Geometry check sheet. Reference: the model listing, model coordinates, mm. Face numbers are marked on the shaded views. A direction names the side the tool comes from. Coordinates: 2 decimals unless noted, no trailing zeros. Write each loop counter-clockwise with the first axis right and the second up, starting at its lowest first coordinate (ties: lowest second). Pieces come first, ordered by that corner, then holes. Notation, with made-up numbers: (-12.5, 75) -> (18.5, 75) arc R7 cw to (18.5, 84) -> close; hole circle Ø5 at (-6.5, -8). An arc over 180 degrees is marked (long way). One line per question, with ' | ' between items.
```python
from build123d import *

# Parameters (mm, degrees)
CUT_EXTRUDE1_DEPTH                 = 65.668384857
CHAMFER1_SIZE                      = 0.34
SOCKET_HEAD_CAP_SCREW1_D           = 6
SOCKET_HEAD_CAP_SCREW1_CBORE_D     = 9.5
SOCKET_HEAD_CAP_SCREW1_CBORE_DEPTH = 6
CUT_EXTRUDE2_DEPTH                 = 45
BOSS_EXTRUDE1_DEPTH                = 5
SKETCH7_R                          = 1.5
BOSS_EXTRUDE2_DEPTH                = 1
REVOLVE3_ANGLE                     = 90
REVOLVE4_ANGLE                     = 90
TAP1_START                         = 4.7999999
TAP1_OUTLINE_R                     = 2.4585
TAP1_DEPTH                         = 7.2000001


# Read off the part's stored shape, not the designer's step: Tap1
with BuildPart() as part:
    # Sketch1 → Revolve1 (revolve)
    with BuildSketch(Plane.XY, mode=Mode.PRIVATE) as revolve1_sk:
        Polygon((0, 29), (12, 29), (12, 7.5), (-50, 7.5), (-50, 17), (-0.8, 17), (-0.8, 16.32), (0, 16.32), align=None)
    revolve(revolve1_sk.sketch.rotate(Axis((-50, 0, 0), (1, 0, 0)), 90), axis=Axis((-50, 0, 0), (1, 0, 0)))

    # Sketch2 → Cut-Extrude1 (cut, through all)
    with BuildSketch(Plane(origin=(0, 0, 0), x_dir=(0, 0, -1), z_dir=(1, 0, 0))):
        with BuildLine():
            Line((14.696938457, 25), (-14.696938457, 25))
            ThreePointArc((-14.696938457, 25), (0, 29), (14.696938457, 25))
        make_face()
        with BuildLine():
            Line((17, 23.494680249), (17, -23.494680249))
            ThreePointArc((17, -23.494680249), (29, 0), (17, 23.494680249))
        make_face()
        with BuildLine():
            Line((14.696938457, -25), (-14.696938457, -25))
            ThreePointArc((-14.696938457, -25), (0, -29), (14.696938457, -25))
        make_face()
        with BuildLine():
            Line((-17, -23.494680249), (-17, 23.494680249))
            ThreePointArc((-17, 23.494680249), (-29, 0), (-17, -23.494680249))
        make_face()
    extrude(amount=CUT_EXTRUDE1_DEPTH, mode=Mode.SUBTRACT)

    # Chamfer1
    chamfer1_edges = [part.edges().sort_by_distance(p)[0] for p in [
        (-50, 0, -17),
    ]]
    chamfer(chamfer1_edges, length=CHAMFER1_SIZE)

    # Socket Head Cap Screw1 (through all)
    with Locations(Plane(origin=(12, 0, 0), x_dir=(0, 0, -1), z_dir=(1, 0, 0))):
        with Locations((-11.25, 19.485571585), (11.25, -19.485571585), (-11.25, -19.485571585), (11.25, 19.485571585)):
            CounterBoreHole(SOCKET_HEAD_CAP_SCREW1_D / 2, SOCKET_HEAD_CAP_SCREW1_CBORE_D / 2, SOCKET_HEAD_CAP_SCREW1_CBORE_DEPTH)

    # Sketch5 → Cut-Extrude2 (cut)
    with BuildSketch(Plane(origin=(0, 0, 0), x_dir=(0, 0, -1), z_dir=(1, 0, 0))):
        with BuildLine():
            Line((-11, -12.961481397), (-11, 12.961481397))
            ThreePointArc((-11, 12.961481397), (-17, 0), (-11, -12.961481397))
        make_face()
    extrude(amount=-CUT_EXTRUDE2_DEPTH, mode=Mode.SUBTRACT)

    # Sketch6 → Boss-Extrude1 (add)
    with BuildSketch(Plane(origin=(0, 0, 11), x_dir=(-1, 0, 0), z_dir=(0, 0, -1))):
        with BuildLine():
            Line((6.5, 4), (36, 4))
            ThreePointArc((36, 4), (40, 0), (36, -4))
            Line((36, -4), (6.5, -4))
            ThreePointArc((6.5, -4), (2.5, 0), (6.5, 4))
        make_face()
    extrude(amount=-BOSS_EXTRUDE1_DEPTH)

    # Sketch7 → Boss-Extrude2 (add)
    with BuildSketch(Plane(origin=(0, 0, 11), x_dir=(-1, 0, 0), z_dir=(0, 0, -1))):
        with Locations(Location((31.821413315, -8.870469014, 0), (0, 0, 180))):
            Circle(SKETCH7_R)
        with Locations(Location((10.678586685, 8.870469014, 0), (0, 0, 180))):
            Circle(SKETCH7_R)
    extrude(amount=-BOSS_EXTRUDE2_DEPTH)

    # Sketch8 → Revolve2 (revolve)
    with BuildSketch(Plane.XY.offset(12)):
        Polygon((-31.821413315, -8.870469014), (-10.678586685, 8.870469014), (-11.642768099, 10.019535678), (-32.78559473, -7.721402349), align=None)
    revolve(axis=Axis((-31.821413315, -8.870469014, 12), (0.7660444431189781, 0.6427876096865394, 0)))

    # Sketch9 → Revolve3 (revolve)
    with BuildSketch(Plane.XY.offset(12)):
        with BuildLine():
            Line((-30.857231901, -10.019535678), (-32.78559473, -7.721402349))
            ThreePointArc((-32.78559473, -7.721402349), (-32.97047998, -9.834650428), (-30.857231901, -10.019535678))
        make_face()
    revolve(axis=Axis((-30.857231901, -10.019535678, 12), (-0.6427876096865415, 0.7660444431189763, 0)), revolution_arc=REVOLVE3_ANGLE)

    # Sketch10 → Revolve4 (revolve)
    with BuildSketch(Plane.XY.offset(12)):
        with BuildLine():
            Line((-11.642768099, 10.019535678), (-9.71440527, 7.721402349))
            ThreePointArc((-9.71440527, 7.721402349), (-9.52952002, 9.834650428), (-11.642768099, 10.019535678))
        make_face()
    revolve(axis=Axis((-11.642768099, 10.019535678, 12), (0.6427876096865339, -0.7660444431189826, 0)), revolution_arc=REVOLVE4_ANGLE)

    # Sketch11 → Cut-Revolve1 (revolve, cut)
    with BuildSketch(Plane.XY, mode=Mode.PRIVATE) as cut_revolve1_sk:
        with BuildLine():
            Line((2.3, 0), (4.8, 0))
            Line((4.8, 0), (4.8, 20.4585))
            ThreePointArc((4.8, 20.4585), (3.032233047, 19.726266953), (2.3, 17.9585))
            Line((2.3, 17.9585), (2.3, 0))
        make_face()
    revolve(cut_revolve1_sk.sketch.rotate(Axis((4.8, 0, 0), (0, 1, 0)), 270), axis=Axis((4.8, 0, 0), (0, 1, 0)), mode=Mode.SUBTRACT)

    # Tap1 outline → Tap1 (cut)
    with BuildSketch(Plane.YZ.offset(TAP1_START)):
        with Locations((18, 0)):
            Circle(TAP1_OUTLINE_R)
    extrude(amount=TAP1_DEPTH, mode=Mode.SUBTRACT)


solid = part.part
```
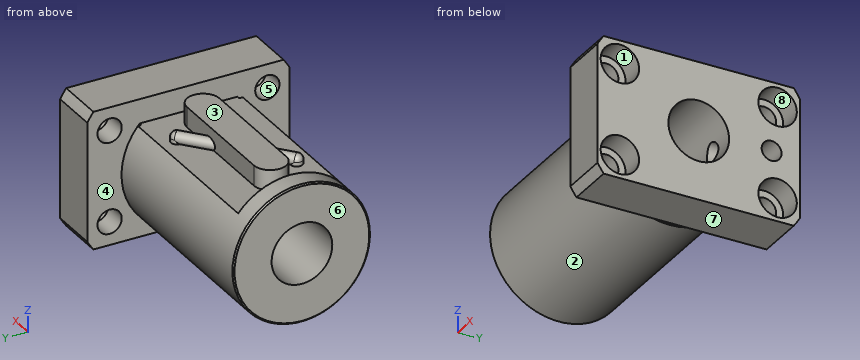
(1) Draft check along Z on the marked faces 5, 6, 7 and 8. Enter one of: pulls with the +Z half, pulls with the -Z half, needs draft (parallel to the pull), parting line crosses it, or undercut.
Answers below:
face 5: undercut | face 6: needs draft | face 7: pulls with the -Z half | face 8: undercut
(2) Cross-section at A-A (y = 0). Record the cut outline in (x, z), plus the area to 3 significant figures.
Answers below:
outline: (-50, -16.66) -> (-49.66, -17) -> (-0.8, -17) -> (-0.8, -16.32) -> (0, -16.32) -> (0, -17) -> (12, -17) -> (12, -7.5) -> (-50, -7.5) -> close; (-50, 7.5) -> (12, 7.5) -> (12, 17) -> (0, 17) -> (0, 11) -> (-2.5, 11) -> (-2.5, 16) -> (-40, 16) -> (-40, 11) -> (-45, 11) -> (-45, 17) -> (-49.66, 17) -> (-50, 16.66) -> close | area: 1,090 mm²
(3) Tool access check on the marked faces 1, 2, 3 and 4. Record the directions out of +Z, -Z, +X, -X, +Y, -Y that give a thin tool (end or side, any length) a straight path to the whole face; none if there is none.
Answers below:
face 1: +X | face 2: -X | face 3: +Z, +Y, -Y | face 4: none
(4) Cross-section at D-D (x = -4). Record the cut outline in (y, z), plus the area to 3 significant figures.
Answers below:
outline: (-12.96, 11) arc R17 ccw (long way) to (12.96, 11) -> (3.12, 11) -> (3.12, 16) -> (-3.12, 16) -> (-3.12, 11) -> close; hole circle Ø15 at (0, 0) | area: 654 mm²
(5) Depth check by flat-ended pin: P1, Ø3, axis at x = -27, y = -7, coming from the -Z side; P2, Ø20.5, axis at x = -28, y = 5.5, coming from the +Z side; P3, Ø8.5, axis at y = -19.49, z = 11.25, coming from the -X side. Enter the tip coordinate at first touch or a pass-through.
Answers below:
P1: stops at z = -16.09 | P2: stops at z = 16 | P3: stops at x = 0
(6) Material ranges on line 1 (Y direction, x = 8, z = 11); line 2 (Y direction, x = 3.95, z = 11.25); line 3 (Z direction, x = 8, y = 18.5), recorded low to high.
Answers below:
line 1: y = -25 to -24.23, -14.74 to 14.74, 24.23 to 25 | line 2: y = -25 to -22.49, -16.49 to 16.49, 22.49 to 25 | line 3: z = -17 to -15.9, -6.6 to -2.41, 2.41 to 6.6, 15.9 to 17
(7) Cross-section at B-B (z = 0). Record the cut outline in (x, y), plus the area to 3 significant figures.
Answers below:
outline: (-50, -16.66) -> (-49.66, -17) -> (-0.8, -17) -> (-0.8, -16.32) -> (0, -16.32) -> (0, -25) -> (12, -25) -> (12, -7.5) -> (-50, -7.5) -> close; (-50, 7.5) -> (2.3, 7.5) -> (2.3, 17.96) arc R2.5 cw to (4.8, 20.46) -> (12, 20.46) -> (12, 25) -> (0, 25) -> (0, 16.32) -> (-0.8, 16.32) -> (-0.8, 17) -> (-49.66, 17) -> (-50, 16.66) -> close; (7.3, 7.5) -> (12, 7.5) -> (12, 15.54) -> (7.3, 15.54) -> close | area: 1,280 mm²
(8) Cross-section at C-C (x = -34.5). Record the cut outline in (y, z), plus the area to 3 significant figures.
Answers below:
outline: (-12.96, 11) arc R17 ccw (long way) to (12.96, 11) -> (4, 11) -> (4, 16) -> (-4, 16) -> (-4, 11) -> close; hole circle Ø15 at (0, 0) | area: 663 mm²
